Read the model definition and answer for the solid it produces. Units are mm, in the model's axes. A direction names the side the tool comes from. Round coordinates to 2 decimals unless told otherwise and drop trailing zeros. Loops run counter-clockwise (first coordinate to the right, second up) from the corner with the lowest first, then second, coordinate; pieces in that order, holes last. Notation, with made-up numbers: (81, 4) -> (138, 4) arc R12 ccw to (138, 19) -> close; hole circle Ø2 at (59.25, 12.25). An arc over 180 degrees is marked (long way). Put each result on its own line as item: value.
Autodesk Inventor part; units mm, degrees
ref_plane "Work Plane1" through (0, 0, 160) normal (0, 0, -1) x (-1, 0, 0)
ref_plane "YZ Plane" through (0, 0, 0) normal (1, 0, 0) x (0, 1, 0)
ref_plane "XZ Plane" through (0, 0, 0) normal (0, 1, 0) x (-1, 0, 0)
sketch "Sketch1" plane through (0, 0, 0) normal (0, 0, 1) x (1, 0, 0)
  line L0 (-15, 15) -> (15, 15)
  line L1 (15, 15) -> (15, -15)
  line L2 (15, -15) -> (-15, -15)
  line L3 (-15, -15) -> (-15, 15)
  line L4 (12.5, 12.5) -> (-12.5, 12.5)
  line L5 (-12.5, 12.5) -> (-12.5, -12.5)
  line L6 (-12.5, -12.5) -> (12.5, -12.5)
  line L7 (12.5, -12.5) -> (12.5, 12.5)
  point P0 (0, 0)
  dimension "d0" = 30
  dimension "d1" = 30
  dimension "d2" = 15
  dimension "d3" = 15
  dimension "d4" = 2.5
extrude "Extrusion1" add sketch "Sketch1" along normal blind 1000
fillet "Fillet1" radius 2 4 edges at (15, 15, 500) (-15, 15, 500) (-15, -15, 500) (15, -15, 500)
ref_plane "Work Plane1" through (0, 0, 160) normal (0, 0, -1) x (-1, 0, 0)
split "Split1" plane through (0, 0, 160) removes the side toward (0, 0, 1)
sketch "Sketch2" plane through (-13, 15, 0) normal (0, 1, 0) x (1, 0, 0)
  point P0 (13, 0)
  point P1 (13, -20)
  dimension "d9" = 0
  dimension "d10" = 20
hole "Hole1" at (0, 15, 20) direction (0, -1, 0) diameter 5 end through all
pattern_linear "Rectangular Pattern1" count 4 spacing 20 along (0, 0, 1) of "Hole1"
sketch "Sketch3" plane through (-13, 15, 0) normal (0, 1, 0) x (1, 0, 0)
  line L0 (0, -160) -> (26, -160)
  point P0 (13, 0)
  point P1 (13, -140)
  point P2 (13, -120)
  dimension "d21" = 20
  dimension "d22" = 0
  dimension "d30" = 0
  dimension "d31" = 20
hole "Hole2" at (0, 15, 140) at (0, 15, 120) direction (0, -1, 0) diameter 5 end through all
equation "\"d0\" = sm_varx_squareBarDimension"
equation "\"d1\" = d0"
equation "\"d4\" = sm_varx_squareBarThickness"
equation "\"d11\" = sm_varx_pinPlate_holeDiameter"
equation "\"d20\" = 0.666667 * sm_varx_squareBarDimension"
equation "\"d23\" = sm_varx_pinPlate_holeDiameter"
equation "\"sm_varx_squareBarDimension\" = 30"
equation "\"sm_varx_squareBarThickness\" = 2.5"
equation "\"sm_varx_pinPlate_holeDiameter\" = 5"
equation "\"hoop_angle_z\" = 45deg"
equation "\"hoop_bearing_length\" = 5deg"
equation "\"hoop_cable_diam\" = 5"
equation "\"hoop_cable_pulley_diam\" = 22"
equation "\"hoop_thickness_large\" = 4"
equation "\"hoop_thickness_medium\" = 3.2"
equation "\"hoop_thickness_small\" = 2"
equation "\"hoop_width_large\" = 51"
equation "\"hoop_width_medium\" = 33.7"
equation "\"hoop_width_small\" = 25.4"
equation "\"rack_tooth_addendum\" = 5"
equation "\"rack_tooth_dedendum\" = 5"
equation "\"rack_tooth_thickness\" = 5"
equation "\"secure_arm_angle\" = 35deg"
equation "\"secure_arm_radii\" = 9"
equation "\"support_baseClamp_platformLengthBuffer\" = 35"
equation "\"support_baseClamp_platformThickness\" = 15"
equation "\"support_baseClamp_platformWidthBuffer\" = 0"
equation "\"support_baseClamp_sleeveHoleDiameter\" = 12"
equation "\"support_baseClamp_sleeveSweepTerminationAngle\" = 55deg"
equation "\"support_baseClamp_thickness\" = 8"
equation "\"support_frame_endHoleBuffer\" = 45"
equation "\"support_frame_squareBarFillet\" = 2"
equation "\"support_frame_squareBarThickness\" = 5"
equation "\"hoop_tabs_thickness\" = 6"
equation "\"hoop_tabs_hole\" = 12"
equation "\"wheelchair_deployed_width\" = 635"
equation "\"wheelchair_deployed_length\" = 1067"
equation "\"wheelchair_deployed_height\" = 914"
equation "\"sm_varx_pinPlate_thickness\" = 5"
equation "\"sm_varx_member_tolerance\" = 0"
equation "\"hoop_bushing12_radialInterference\" = 0"
equation "\"hoop_bushing23_radialInterference\" = 0"
equation "\"hoop_bushing23_od\" = -2 * hoop_thickness_medium + hoop_width_medium + hoop_bushing23_radialInterference"
equation "\"hoop_bushing23_thickness\" = -hoop_width_small + hoop_bushing23_od - 2 * hoop_bushing23_radialInterference"
equation "\"hoop_bushing12_od\" = -2 * hoop_thickness_large + hoop_width_large + hoop_bushing12_radialInterference"
equation "\"wheelchatir_pos_deploy_angle_0\" = 65deg"
equation "\"wheelchatir_pos_store_angle_0\" = 90deg"
equation "\"wheelchatir_pos_deploy_angle_1\" = 20deg"
equation "\"wheelchatir_pos_store_angle_1\" = 20deg"
equation "\"hoop_bushing12_thickness\" = -hoop_width_medium + hoop_bushing12_od - 2 * hoop_bushing12_radialInterference"
properties part number "member_vertical" material "Steel, Galvanized"
Item 1: The part is cut by section A-A (x = -8). Determine the outline of the cut face in (y, z), then the cut area to 3 significant figures.
Derived:
outline: (-15, 0) -> (-12.5, 0) -> (-12.5, 160) -> (-15, 160) -> close; (12.5, 0) -> (15, 0) -> (15, 160) -> (12.5, 160) -> close
area: 800 mm^2
Item 2: The part is cut by section D-D (z = 29). Determine the outline of the cut face in (x, y).
Derived:
outline: (-15, -13) arc R2 ccw to (-13, -15) -> (13, -15) arc R2 ccw to (15, -13) -> (15, 13) arc R2 ccw to (13, 15) -> (-13, 15) arc R2 ccw to (-15, 13) -> close; hole (-12.5, -12.5) -> (12.5, -12.5) -> (12.5, 12.5) -> (-12.5, 12.5) -> close
Item 3: A flat-ended cylindrical pin translates along its axis: pin 1 Ø4.5 at (x, z) = (0, 80) entering from +Y. Find the tip coordinate at first contact, or state that the pin passes through.
Derived:
pin 1: passes through
Item 4: Which of the six approach directions +Z, -Z, +X, -X, +Y, -Y give full straight-line access (tool end or side, diameter ignored) to faces 4 (the flat face through (3, 12.5, 79)), 5 (the cylindrical face through (0.96, 13.73, 62.31))?
Derived:
face 4: +Z, -Z
face 5: +Y, -Y
Item 5: Find the intervals of material crossed by line 1 along Y through (x, z) = (-8.25, 93); line 2 along X through (y, z) = (13.35, 20), in increasing order.
Derived:
line 1: y = -15 to -12.5, 12.5 to 15
line 2: x = -14.97 to -2.5, 2.5 to 14.97
Item 6: For a pull along X with two mould halves and no side action, classify faces 1 (the flat face through (3, -15, 79)), 2 (the flat face through (-15, 0, 79)), 3 (the cylindrical face through (-0.1, 13.7, 77.5)) as pulls with the +X half, pulls with the -X half, needs draft (parallel to the pull), parting line crosses it, or undercut.
Derived:
face 1: needs draft
face 2: pulls with the -X half
face 3: undercut
Item 7: The part is cut by section B-B (z = 60). Determine the outline of the cut face in (x, y), then the cut area to 3 significant figures.
Derived:
outline: (-15, -13) arc R2 ccw to (-13, -15) -> (-2.5, -15) -> (-2.5, -12.5) -> (-12.5, -12.5) -> (-12.5, 12.5) -> (-2.5, 12.5) -> (-2.5, 15) -> (-13, 15) arc R2 ccw to (-15, 13) -> close; (2.5, -15) -> (13, -15) arc R2 ccw to (15, -13) -> (15, 13) arc R2 ccw to (13, 15) -> (2.5, 15) -> (2.5, 12.5) -> (12.5, 12.5) -> (12.5, -12.5) -> (2.5, -12.5) -> close
area: 247 mm^2
